Input: part model. Units: mm. Frame: model coordinates. A direction names the side the tool comes from. Round coordinates to 2 decimals unless told otherwise and drop trailing zeros. Write each loop counter-clockwise with the first axis right and the second up, starting at its lowest first coordinate (ties: lowest second). Pieces come first, ordered by that corner, then holes. Notation, with made-up numbers: (86.5, 39) -> (130.5, 39) arc R24 ccw to (130.5, 71) -> close; hole circle Ø6 at (52.5, 66). An arc over 180 degrees is marked (long way). Write item = value, one per line.
```python
from build123d import *

# Parameters (mm, degrees)
BOSS_EXTRUDE1_DEPTH = 3.175
CUT_EXTRUDE1_DEPTH  = 3.175
LPATTERN1_COUNT     = 25
LPATTERN1_PITCH     = 6


with BuildPart() as part:
    # Sketch1 → Boss-Extrude1 (new body)
    with BuildSketch(Plane(origin=(0, 0, 0), x_dir=(1, 0, 0), z_dir=(0, 1, 0))):
        with BuildLine():
            Line((-6.35, 0), (-56.134, 0))
            ThreePointArc((-56.134, 0), (-59.309, -3.175), (-56.134, -6.35))
            Line((-56.134, -6.35), (56.134, -6.35))
            ThreePointArc((56.134, -6.35), (59.309, -3.175), (56.134, 0))
            Line((56.134, 0), (6.35, 0))
            Line((6.35, 0), (6.35, 152.4))
            Line((6.35, 152.4), (-6.35, 152.4))
            Line((-6.35, 152.4), (-6.35, 0))
        make_face()
    extrude(amount=BOSS_EXTRUDE1_DEPTH)

    # Sketch2 → Cut-Extrude1 (cut)
    with BuildSketch(Plane(origin=(0, 3.175, 0), x_dir=(1, 0, 0), z_dir=(0, 1, 0))):
        Polygon((-6.35, 150.4), (-4.869501466, 149.4), (-4.869501466, 147.4), (-6.35, 146.4), align=None)
    cut_extrude1 = extrude(amount=-CUT_EXTRUDE1_DEPTH, mode=Mode.SUBTRACT)

    # LPattern1: Cut-Extrude1 ×25
    with Locations(*[(0, 0, i * LPATTERN1_PITCH) for i in range(1, LPATTERN1_COUNT)]):
        add(cut_extrude1, mode=Mode.SUBTRACT)


solid = part.part
```
1) Access query for faces 1 (the face through (6.35, 2, -75)), 2 (the face through (-1, 2, 6.35)), 3 (the face through (-31, 2, 0)). Directions: +Z, -Z, +X, -X, +Y, -Y. A direction counts if a zero-diameter tool reaches every point of the face in a straight line with its end or side. Return the directions, or none.
Solutions:
face_1 = -Z, +X, +Y, -Y
face_2 = +Z, +X, -X, +Y, -Y
face_3 = -Z, -X, +Y, -Y
2) Line query: L1, parallel to X at y = 0.6, z = -16; L2, parallel to Z at x = -40.5, y = 2.95. Output: solid intervals per line, ascending. Write a range as from..to.
Solutions:
L1 = -4.87..6.35
L2 = 0..6.35
3) First-contact query: P1, Ø0.6, axis at y = 1, z = -4.5, coming from the -X side; P2, Ø1, axis at y = 2, z = -133, coming from the +X side; P3, Ø1, axis at y = 2.5, z = -31, coming from the -X side. Flat tips, straight axial feed; report the tip coordinate or a pass-through.
Solutions:
P1 = -4.87
P2 = 6.35
P3 = -6.35
4) Cut plane A-A (x = 33.5). Return the cut outline in (y, z) (3 decimals), and give its area (3 significant figures).
Solutions:
outline = (0, 0) -> (3.175, 0) -> (3.175, 6.35) -> (0, 6.35) -> close
area = 20.2 mm^2
